```python
from build123d import *

# Parameters (mm, degrees)
SKETCH1_R           = 7
SKETCH1_R_2         = 4
SKETCH1_RX          = 62
SKETCH1_RY          = 13.5
BOSS_EXTRUDE3_DEPTH = 2


with BuildPart() as part:
    # Sketch1 → Boss-Extrude3 (new body)
    # profile 1 of 3: a face of its own
    with BuildSketch(Plane.XY):
        Circle(SKETCH1_R)
        Circle(SKETCH1_R_2, mode=Mode.SUBTRACT)
    # profile 2 of 3: a face of its own
    with BuildSketch(Plane.XY):
        with Locations(Location((0, 68), (0, 0, 90))):
            Ellipse(SKETCH1_RX, SKETCH1_RY)
    # profile 3 of 3: a face of its own
    with BuildSketch(Plane.XY):
        with Locations(Location((0, -68), (0, 0, -90))):
            Ellipse(SKETCH1_RX, SKETCH1_RY)
    extrude(amount=BOSS_EXTRUDE3_DEPTH)


solid = part.part
```
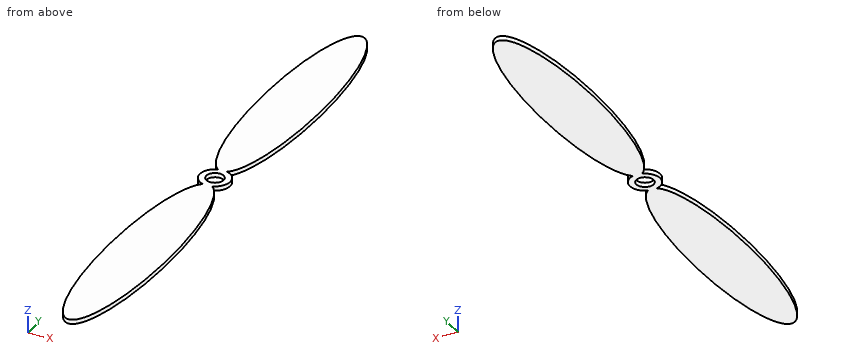
The model under review builds one solid part; all positions refer to its coordinate system, in mm. Coordinates: 2 decimals unless noted, no trailing zeros. Write each loop counter-clockwise with the first axis right and the second up, starting at its lowest first coordinate (ties: lowest second). Pieces come first, ordered by that corner, then holes. Notation, with made-up numbers: (66.5, 18) -> (125.5, 18) arc R19 ccw to (125.5, 48) -> close; hole circle Ø3 at (16.5, -31). An arc over 180 degrees is marked (long way). One line per item, written item: value. Start each with the question number.
Q1. To check wall thickness, follow probe 1 along Y at (x, z) = (4.25, 1.1); probe 2 along Y at (x, z) = (-4.75, 1); probe 3 along Y at (x, z) = (1.75, 1.5). State the ranges of each line that lie inside material, in increasing order.
Q2. Add section A-A, the plane y = 0. Give the boundary of the cut face in (x, z), then the cut area to 3 significant figures.
Q3. Clearance check with flat-ended pins moving along their axes: P1, Ø5, axis at x = 0, y = 0, coming from the +Z side; P2, Ø3, axis at x = 8.5, y = -81, coming from the -Z side; P3, Ø1, axis at y = 26, z = 0, coming from the -X side. State where each tip first meets the part, or that it passes through.
Response:
1. probe 1: -126.85 to -9.15, -5.56 to 5.56, 9.15 to 126.85
1. probe 2: -126.04 to -9.96, -5.14 to 5.14, 9.96 to 126.04
1. probe 3: -129.48 to -3.6, 3.6 to 129.48
2. outline: (-7, 0) -> (-4, 0) -> (-4, 2) -> (-7, 2) -> close; (4, 0) -> (7, 0) -> (7, 2) -> (4, 2) -> close
2. area: 12.0 mm²
3. P1: through
3. P2: z = 0
3. P3: x = -10.03
